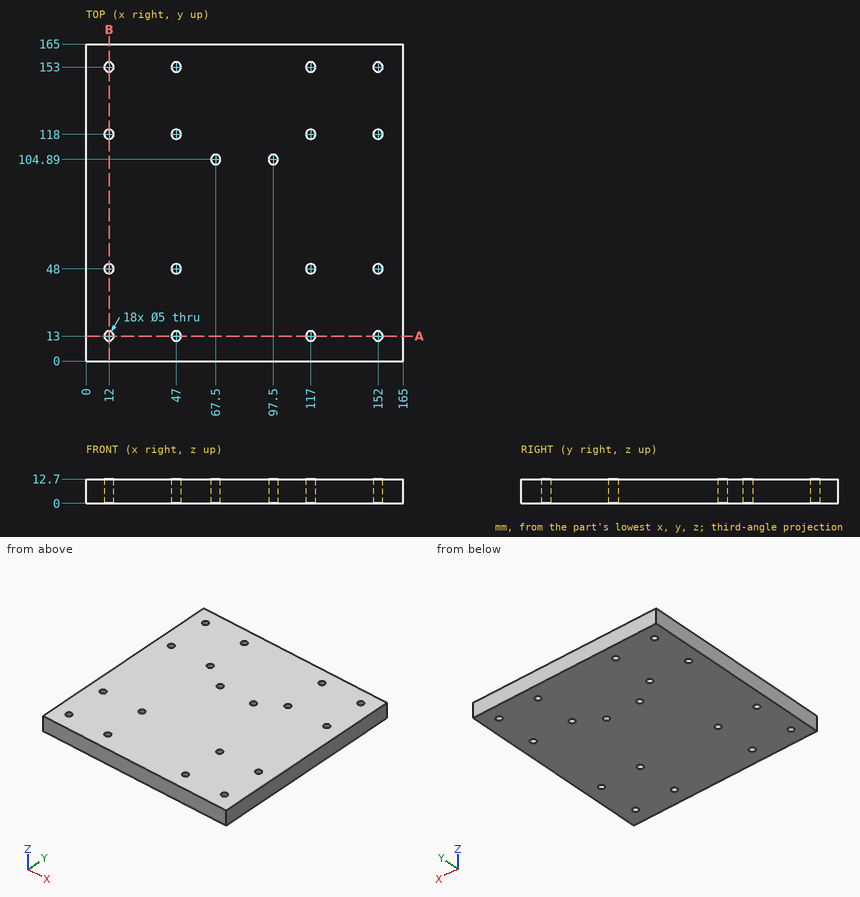
Source: three-view drawing plus pictorial views. Frame: mm from the lowest corner of the part. Coordinates: 2 decimals unless noted, no trailing zeros. Order: outer loops, then holes, each group sorted by start corner. A loop starts at its lowest first (then second) coordinate and runs counter-clockwise, first axis right, second up.
Item 1: Cut plane B-B (x = 12). Return loops of the section in (y, z).
Output values:
outline: (0, 0) - (10.5, 0) - (10.5, 12.7) - (0, 12.7) - close; (15.5, 0) - (45.5, 0) - (45.5, 12.7) - (15.5, 12.7) - close; (50.5, 0) - (115.5, 0) - (115.5, 12.7) - (50.5, 12.7) - close; (120.5, 0) - (150.5, 0) - (150.5, 12.7) - (120.5, 12.7) - close; (155.5, 0) - (165, 0) - (165, 12.7) - (155.5, 12.7) - close
Item 2: Material intervals for line 1 (X direction, y = 153, z = 7.75); line 2 (Y direction, x = 47, z = 7.5); line 3 (Y direction, x = 45, z = 9), sorted ascending.
Output values:
line 1: x = 0 to 9.5, 14.5 to 44.5, 49.5 to 114.5, 119.5 to 149.5, 154.5 to 165
line 2: y = 0 to 10.5, 15.5 to 45.5, 50.5 to 115.5, 120.5 to 150.5, 155.5 to 165
line 3: y = 0 to 11.5, 14.5 to 46.5, 49.5 to 116.5, 119.5 to 151.5, 154.5 to 165
Item 3: Cut plane A-A (y = 13). Return loops of the section in (x, z).
Output values:
outline: (0, 0) - (9.5, 0) - (9.5, 12.7) - (0, 12.7) - close; (14.5, 0) - (44.5, 0) - (44.5, 12.7) - (14.5, 12.7) - close; (49.5, 0) - (114.5, 0) - (114.5, 12.7) - (49.5, 12.7) - close; (119.5, 0) - (149.5, 0) - (149.5, 12.7) - (119.5, 12.7) - close; (154.5, 0) - (165, 0) - (165, 12.7) - (154.5, 12.7) - close
